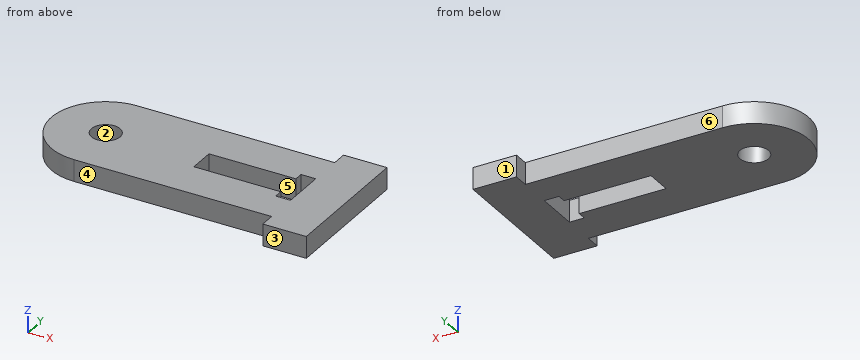
from build123d import *

# Parameters (mm, degrees)
SKETCH1_R           = 1.65
SKETCH1_W           = 10
SKETCH1_H           = 12.5
BOSS_EXTRUDE1_DEPTH = 2.5
SKETCH2_W           = 5
SKETCH2_H           = 16
BOSS_EXTRUDE2_DEPTH = 2.5
SKETCH3_W           = 1.7
SKETCH3_H           = 5
CUT_EXTRUDE1_DEPTH  = 29.940283343
SKETCH5_W           = 10
SKETCH5_H           = 3
CUT_EXTRUDE2_DEPTH  = 29.940283343


with BuildPart() as part:
    # Sketch1 → Boss-Extrude1 (new body)
    # profile 1 of 2: a face of its own
    with BuildSketch(Plane.XY):
        with BuildLine():
            ThreePointArc((0, 6.25), (-6.25, 0), (0, -6.25))
            Line((0, -6.25), (12.7, -6.25))
            Line((12.7, -6.25), (12.7, 6.25))
            Line((12.7, 6.25), (0, 6.25))
        make_face()
        Circle(SKETCH1_R, mode=Mode.SUBTRACT)
    # profile 2 of 2: a face of its own
    with BuildSketch(Plane.XY):
        with Locations((17.7, 0)):
            Rectangle(SKETCH1_W, SKETCH1_H)
    extrude(amount=BOSS_EXTRUDE1_DEPTH)

    # Sketch2 → Boss-Extrude2 (add)
    with BuildSketch(Plane.XY.offset(2.5)):
        with Locations((25.2, 0)):
            Rectangle(SKETCH2_W, SKETCH2_H)
    extrude(amount=-BOSS_EXTRUDE2_DEPTH)

    # Sketch3 → Cut-Extrude1 (cut, through all)
    with BuildSketch(Plane.XY.offset(2.5)):
        with Locations((21.85, 0)):
            Rectangle(SKETCH3_W, SKETCH3_H)
    extrude(amount=-CUT_EXTRUDE1_DEPTH, mode=Mode.SUBTRACT)

    # Sketch5 → Cut-Extrude2 (cut, through all)
    with BuildSketch(Plane.XY.offset(2.5)):
        with Locations((16, 0)):
            Rectangle(SKETCH5_W, SKETCH5_H)
    extrude(amount=-CUT_EXTRUDE2_DEPTH, mode=Mode.SUBTRACT)


solid = part.part
The listing builds one solid part. Answer for the finished solid, in the listing's coordinates (mm). Face numbers are marked on the shaded views. A direction names the side the tool comes from. Give positions to 0.01 mm unless a question says otherwise; leave off trailing zeros. Loops run counter-clockwise (first coordinate to the right, second up) from the corner with the lowest first, then second, coordinate; pieces in that order, holes last. Notation, with made-up numbers: (-21, -35) - (-6, -35) arc R27 ccw to (-6, -18) - close; hole circle Ø8 at (-26.5, 69.5). An arc over 180 degrees is marked (long way). Answer as a JSON object with one key per item and string values.
1. Flat-ended cylindrical pins translate along their axes: pin 1 Ø1 at (x, z) = (3, 2) entering from +Y; pin 2 Ø0.9 at (x, z) = (22, 1) entering from -Y; pin 3 Ø0.9 at (y, z) = (-7.5, 1.5) entering from -X. Find the tip coordinate at first contact, or state that the pin passes through.
Determined:
{"pin 1": "y = 6.25", "pin 2": "y = -6.25", "pin 3": "x = 22.7"}
2. A cutting plane is placed at B-B (y = 0). Write down the section's boundary in (x, z), then the cut area to 3 significant figures.
Determined:
{"outline": "(-6.25, 0) - (-1.65, 0) - (-1.65, 2.5) - (-6.25, 2.5) - close; (1.65, 0) - (11, 0) - (11, 2.5) - (1.65, 2.5) - close; (22.7, 0) - (27.7, 0) - (27.7, 2.5) - (22.7, 2.5) - close", "area": "47.4 mm²"}
3. A cutting plane is placed at D-D (y = -5). Write down the section's boundary in (x, z).
Determined:
{"outline": "(-3.75, 0) - (27.7, 0) - (27.7, 2.5) - (-3.75, 2.5) - close"}
4. For a pull along Y with two mould halves and no side action, classify the marked faces 1, 2 and 3 as pulls with the +Y half, pulls with the -Y half, needs draft (parallel to the pull), parting line crosses it, or undercut.
Determined:
{"face 1": "pulls with the +Y half", "face 2": "undercut", "face 3": "pulls with the -Y half"}
5. A cutting plane is placed at A-A (x = 17). Write down the section's boundary in (y, z).
Determined:
{"outline": "(-6.25, 0) - (-1.5, 0) - (-1.5, 2.5) - (-6.25, 2.5) - close; (1.5, 0) - (6.25, 0) - (6.25, 2.5) - (1.5, 2.5) - close"}
6. A cutting plane is placed at C-C (z = 1.1). Write down the section's boundary in (x, y).
Determined:
{"outline": "(0, -6.25) - (22.7, -6.25) - (22.7, -8) - (27.7, -8) - (27.7, 8) - (22.7, 8) - (22.7, 6.25) - (0, 6.25) arc R6.25 ccw to start; hole circle Ø3.3 at (0, 0); hole (11, -1.5) - (21, -1.5) - (21, -2.5) - (22.7, -2.5) - (22.7, 2.5) - (21, 2.5) - (21, 1.5) - (11, 1.5) - close"}
7. Find the intervals of material crossed by L1, parallel to Y at x = 0, z = 1.4; L2, parallel to Y at x = 14, z = 0.9; L3, parallel to X at y = -1.25, z = 0.35, in increasing order. Write a range as [from, to].
Determined:
{"L1": "[-6.25, -1.65], [1.65, 6.25]", "L2": "[-6.25, -1.5], [1.5, 6.25]", "L3": "[-6.12, -1.08], [1.08, 11], [22.7, 27.7]"}
8. For the marked faces 4, 5 and 6, determine the directions among +Z, -Z, +X, -X, +Y, -Y from which every point of the face is accessible in a straight line to the end or side of a thin tool.
Determined:
{"face 4": "+Z, -Z, -X, -Y", "face 5": "+Z, -Z", "face 6": "+Z, -Z, -X, +Y"}
